Part model, mm, in its own coordinate system. Face numbers are marked on the shaded views. Coordinates: 2 decimals unless noted, no trailing zeros. Loops run counter-clockwise (first coordinate to the right, second up) from the corner with the lowest first, then second, coordinate; pieces in that order, holes last. Notation, with made-up numbers: (21, 12) -> (59, 12) arc R25 cw to (59, 42) -> close; hole circle Ø1 at (-36.75, 51.5). An arc over 180 degrees is marked (long way). Use one line per item in the form item = value. Start each with the question number.
(1) Mould opens along Y. For the marked faces 1, 2, 3 and 4 say: +Y half, -Y half, draft (parallel to the pull), parting line (faces both ways), or undercut.
(2) Band-saw the part on A-A on y = -1. Give the cut face in (x, z).
(3) Band-saw the part on D-D on z = 7. Give the cut face in (x, y) (3 decimals), then the cut area to 3 significant figures.
(4) Pin check, flat tips, straight feed: P1, Ø10, axis at x = 26.5, y = -1, coming from the -Z side; P2, Ø1, axis at y = 10, z = 1.5, coming from the +X side; P3, Ø2, axis at y = 6, z = 6, coming from the -X side. Stop position of each tip, or through.
(5) Band-saw the part on C-C on x = 26. Give the cut face in (y, z).
(6) Drill centre lines: L1, parallel to X at y = 1.5, z = 4.75; L2, parallel to Y at x = 15.5, z = 5.5; L3, parallel to X at y = -14, z = 7. Where is each one in solid material? Low to high. Write a range as [from, to].
(7) Band-saw the part on B-B on x = 36. Give the cut face in (y, z), then the cut area to 3 significant figures.
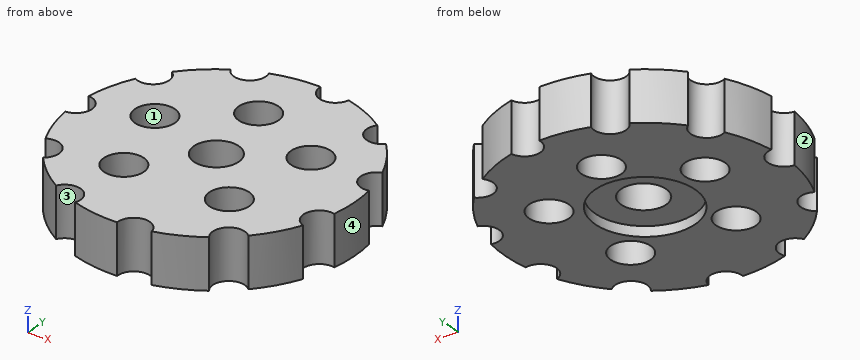
```python
from build123d import *

# Parameters (mm, degrees)
CYLINDER009_R      = 3.2
CYLINDER009_DEPTH  = 10
ARRAY001_COUNT     = 11
CYLINDER010_R      = 28.02
CYLINDER010_DEPTH  = 10
SKETCH002_R        = 4.5
SKETCH002_R_2      = 4
POCKET001_DEPTH    = 10.001
SKETCH003_R        = 10
POCKET002002_DEPTH = 2


with BuildPart() as obj1:
    # Cylinder009 → Cylinder009 (new body)
    with BuildSketch(Plane.XY):
        Circle(CYLINDER009_R)
    extrude(amount=CYLINDER009_DEPTH)

    # Array001: obj1 ×11 about axis
    array001_axis = Axis((28.02, 0, 0), (0, 0, 1))


with BuildPart() as obj1_1:
    add(obj1.part)
    for i in range(1, ARRAY001_COUNT):
        add(obj1.part.rotate(array001_axis, i * 360 / ARRAY001_COUNT))


with BuildPart() as taladro_servohorn:
    # Cylinder010 → Cylinder010 (new body)
    with BuildSketch(Plane(origin=(28.02, 0, 0), x_dir=(1, 0, 0), z_dir=(0, 0, 1))):
        Circle(CYLINDER010_R)
    extrude(amount=CYLINDER010_DEPTH)

    # Cut007: cut obj1
    add(obj1_1.part, mode=Mode.SUBTRACT)

    # Sketch002 → Pocket001 (cut, through all)
    with BuildSketch(Plane.XY.offset(10)):
        with Locations((28.352856, -0.047906)):
            Circle(SKETCH002_R)
        with Locations((18.376312, -11.904833)):
            Circle(SKETCH002_R_2)
        with Locations((41.523029, 8.031758)):
            Circle(SKETCH002_R_2)
        with Locations((38.98872, -10.975584)):
            Circle(SKETCH002_R_2)
        with Locations((12.800824, 4.230289)):
            Circle(SKETCH002_R_2)
        with Locations((25.88417, 14.927018)):
            Circle(SKETCH002_R_2)
    extrude(amount=-POCKET001_DEPTH, mode=Mode.SUBTRACT)

    # Sketch003 → Pocket002002 (cut)
    with BuildSketch(Plane(origin=(0, 0, 0), x_dir=(1, 0, 0), z_dir=(0, 0, -1))):
        with Locations((28.02, 0.027806)):
            Circle(SKETCH003_R)
    extrude(amount=-POCKET002002_DEPTH, mode=Mode.SUBTRACT)


solid = taladro_servohorn.part
```
A:
q1.face_1 = undercut
q1.face_2 = -Y half
q1.face_3 = undercut
q1.face_4 = parting line
q2.outline = (3.04, 0) -> (18.07, 0) -> (18.07, 2) -> (23.95, 2) -> (23.95, 10) -> (3.04, 10) -> close; (32.75, 2) -> (37.97, 2) -> (37.97, 0) -> (56.02, 0) -> (56.02, 10) -> (32.75, 10) -> close
q3.outline = (0.183, -3.195) arc R28.02 ccw to (2.875, -12.362) arc R3.2 cw to (6.329, -17.738) arc R28.02 ccw to (13.55, -23.995) arc R3.2 cw to (19.362, -26.649) arc R28.02 ccw to (28.819, -28.009) arc R3.2 cw to (35.144, -27.099) arc R28.02 ccw to (43.835, -23.13) arc R3.2 cw to (48.664, -18.946) arc R28.02 ccw to (53.83, -10.908) arc R3.2 cw to (55.63, -4.777) arc R28.02 ccw to (55.63, 4.777) arc R3.2 cw to (53.83, 10.908) arc R28.02 ccw to (48.664, 18.946) arc R3.2 cw to (43.835, 23.13) arc R28.02 ccw to (35.144, 27.099) arc R3.2 cw to (28.819, 28.009) arc R28.02 ccw to (19.362, 26.649) arc R3.2 cw to (13.55, 23.995) arc R28.02 ccw to (6.329, 17.738) arc R3.2 cw to (2.875, 12.362) arc R28.02 ccw to (0.183, 3.195) arc R3.2 cw to start; hole circle Ø8 at (12.801, 4.23); hole circle Ø8 at (18.376, -11.905); hole circle Ø8 at (25.884, 14.927); hole circle Ø9 at (28.353, -0.048); hole circle Ø8 at (38.989, -10.976); hole circle Ø8 at (41.523, 8.032)
q3.area = 1,980 mm²
q4.P1 = 2
q4.P2 = 53.05
q4.P3 = 0.45
q5.outline = (-27.95, 0) -> (-9.82, 0) -> (-9.82, 2) -> (-3.88, 2) -> (-3.88, 10) -> (-27.95, 10) -> close; (3.79, 2) -> (9.77, 2) -> (9.77, 0) -> (10.93, 0) -> (10.93, 10) -> (3.79, 10) -> close; (18.93, 0) -> (27.95, 0) -> (27.95, 10) -> (18.93, 10) -> close
q6.L1 = [2.83, 9.88], [15.72, 24.13], [32.58, 56]
q6.L2 = [-22.41, -14.68], [-9.13, 1.28], [7.18, 22.41]
q6.L3 = [7.43, 14.97], [21.78, 36.37], [41.61, 52.29]
q7.outline = (-26.86, 0) -> (-13.63, 0) -> (-13.63, 10) -> (-26.86, 10) -> close; (-8.32, 0) -> (-6.05, 0) -> (-6.05, 2) -> (6, 2) -> (6, 0) -> (26.86, 0) -> (26.86, 10) -> (-8.32, 10) -> close
q7.area = 460 mm²
